Read the model definition and answer for the solid it produces. Units are mm, in the model's axes. A direction names the side the tool comes from. Coordinates: 2 decimals unless noted, no trailing zeros. Write each loop counter-clockwise with the first axis right and the second up, starting at its lowest first coordinate (ties: lowest second). Pieces come first, ordered by that corner, then holes. Notation, with made-up numbers: (64.25, -14.75) -> (73.25, -14.75) arc R22 ccw to (73.25, -3.75) -> close; hole circle Ø2 at (36.25, -22). An arc over 180 degrees is marked (long way). One line per item, written item: value. Start each with the question number.
1. Find section D-D, the plane z = 10. Write down the section's boundary in (x, y), and give its area (3 significant figures).
2. Given P1, Ø4, axis at x = 0, z = 7.5, coming from the -Y side; P2, Ø1, axis at x = -2, z = 5, coming from the +Y side; P3, Ø6, axis at y = 5.5, z = 2, coming from the -X side, each flat-ended and moving along its own axis, determine where each tip first touches the part or whether it passes through.
3. Find section B-B, the plane x = 3. Write down the section's boundary in (y, z).
4. Find section A-A, the plane y = -2.5. Write down the section's boundary in (x, z), and give its area (3 significant figures).
5. For faces 4 (the flat face through (3.5, 8.2, 4)), 5 (the cylindrical face through (2.18, 2.42, 5.42)), determine the directions among +Z, -Z, +X, -X, +Y, -Y from which every point of the face is accessible in a straight line to the end or side of a thin tool.
6. Consider line 1 along Y through (x, z) = (0, 7.5); line 2 along X through (y, z) = (-1, 1); line 3 along X through (y, z) = (-2.25, 3.25). Determine where each line is inside the solid, lowest interval first.
7. For a pull along Y with two mould halves and no side action, classify faces 1 (the cylindrical face through (-1.82, 8.81, 7.45)), 2 (the cylindrical face through (-3.1, -0.2, 5.4)), 3 (the flat face through (0, 2, 11)) as pulls with the +Y half, pulls with the -Y half, needs draft (parallel to the pull), parting line crosses it, or undercut.
8. Find section C-C, the plane x = 6.5. Write down the section's boundary in (y, z), and give its area (3 significant figures).
Autodesk Inventor part; units mm, degrees
ref_plane "YZ Plane" through (0, 0, 0) normal (1, 0, 0) x (0, 1, 0)
ref_plane "XZ Plane" through (0, 0, 0) normal (0, 1, 0) x (-1, 0, 0)
ref_plane "XY Plane" through (0, 0, 0) normal (0, 0, 1) x (1, 0, 0)
sketch "Sketch3" plane through (0, 0, 0) normal (0, 0, 1) x (1, 0, 0)
  circle A0 centre (-0.1954, 1.4872) radius 10
  circle A1 centre (0.5933, 0.2945) radius 7.5 construction
  circle A2 centre (-2.7432, -1.9118) radius 1.75 construction
  circle A3 centre (-2.7432, -1.9118) radius 1.75
  circle A4 centre (3.9298, 2.5008) radius 1.75
  circle A5 centre (3.9298, 2.5008) radius 1.75 construction
  line L0 (3.9298, 2.5008) -> (-2.7432, -1.9118) construction
  line L1 (0.5933, 0.2945) -> (-1.1822, 2.9794) construction
  point P0 (0, 0)
  dimension "d1" = 1.5
  dimension "d2" = 20
  dimension "d9" = 8
extrude "Extrusion1" add sketch "Sketch3" along normal blind 4
sketch "Sketch4" plane through (-0.1954, 1.4872, 4) normal (0, 0, 1) x (1, 0, 0)
  circle A0 centre (0, 0) radius 10 construction
  circle A1 centre (4.1252, 1.0136) radius 1.75 construction
  circle A2 centre (-2.5478, -3.399) radius 1.75 construction
  circle A3 centre (0, 0) radius 7.5
  circle A4 centre (4.1252, 1.0136) radius 1.75
  circle A5 centre (-2.5478, -3.399) radius 1.75
  point P0 (0.1954, -1.4872)
  dimension "d6" = 15
extrude "Extrusion2" add sketch "Sketch4" along normal blind 7
properties part number "Shaft-2"
Answer block:
1. outline: circle Ø15 at (-0.2, 1.49); hole circle Ø3.5 at (-2.74, -1.91); hole circle Ø3.5 at (3.93, 2.5)
1. area: 157 mm2
2. P1: stops at y = -6.01
2. P2: stops at y = 8.87
2. P3: stops at x = -10.14
3. outline: (-7.99, 0) -> (1.02, 0) -> (1.02, 11) -> (-5.3, 11) -> (-5.3, 4) -> (-7.99, 4) -> close; (3.98, 0) -> (10.96, 0) -> (10.96, 4) -> (8.27, 4) -> (8.27, 11) -> (3.98, 11) -> close
4. outline: (-9.37, 0) -> (-4.39, 0) -> (-4.39, 11) -> (-6.55, 11) -> (-6.55, 4) -> (-9.37, 4) -> close; (-1.1, 0) -> (8.98, 0) -> (8.98, 4) -> (6.16, 4) -> (6.16, 11) -> (-1.1, 11) -> close
4. area: 126 mm2
5. face 4: +Z
5. face 5: +Z, -Z
6. line 1: y = -6.01 to 8.98
6. line 2: x = -9.88 to -4.24, -1.25 to 9.49
6. line 3: x = -9.47 to -4.46, -1.03 to 9.08
7. face 1: parting line crosses it
7. face 2: undercut
7. face 3: needs draft
8. outline: (-5.94, 0) -> (8.91, 0) -> (8.91, 4) -> (4.87, 4) -> (4.87, 11) -> (-1.89, 11) -> (-1.89, 4) -> (-5.94, 4) -> close
8. area: 107 mm2
